Work out the finished part from the listing and answer in its coordinate system (mm). A direction names the side the tool comes from. Round coordinates to 2 decimals unless told otherwise and drop trailing zeros. Loops run counter-clockwise (first coordinate to the right, second up) from the corner with the lowest first, then second, coordinate; pieces in that order, holes last. Notation, with made-up numbers: (-30.75, -40) -> (14.25, -40) arc R11 cw to (14.25, -23) -> close; hole circle Ø1 at (1.25, -37.5). An arc over 180 degrees is marked (long way). Use one line per item in the form item = value.
```python
from build123d import *

# Parameters (mm, degrees)
SKICA2_W                 = 20
SKICA2_H                 = 42.3
P_IDAT_VYSUNUT_M1_DEPTH  = 4
SKICA3_W                 = 24
SKICA3_H                 = 42.3
P_IDAT_VYSUNUT_M2_DEPTH  = 4
SKICA4_W                 = 6
SKICA4_H                 = 42.3
P_IDAT_VYSUNUT_M3_DEPTH  = 42.3
SKICA5_R                 = 11.05
ODEBRAT_VYSUNUT_M1_DEPTH = 7
SKICA7_R                 = 2.6
ODEBRAT_VYSUNUT_M3_DEPTH = 4
ZKOSEN_1_SIZE            = 1
SKICA8_W                 = 20
SKICA8_H                 = 4
P_IDAT_VYSUNUT_M4_DEPTH  = 20.091596743
SKICA9_R                 = 2.6
ODEBRAT_VYSUNUT_M4_DEPTH = 4
ODEBRAT_VYSUNUT_M5_DEPTH = 80
SKICA11_W                = 84.692176523
SKICA11_H                = 80.474242756
ODEBRAT_VYSUNUT_M6_DEPTH = 24
SKICA12_W                = 6
SKICA12_H                = 6
SKICA12_H_2              = 10
P_IDAT_VYSUNUT_M5_DEPTH  = 8
SKICA13_R                = 1.6
ODEBRAT_VYSUNUT_M7_DEPTH = 15
SKICA14_W                = 5
SKICA14_H                = 3
ODEBRAT_VYSUNUT_M8_DEPTH = 15


with BuildPart() as part:
    # Skica2 → Přidat vysunutím1 (new body)
    with BuildSketch(Plane.XY):
        with Locations((-14.524287798, -61.15)):
            Rectangle(SKICA2_W, SKICA2_H)
    extrude(amount=P_IDAT_VYSUNUT_M1_DEPTH)

    # Skica3 → Přidat vysunutím2 (add)
    with BuildSketch(Plane.ZY.offset(24.524287798)):
        with Locations((-8, -61.15)):
            Rectangle(SKICA3_W, SKICA3_H)
    extrude(amount=P_IDAT_VYSUNUT_M2_DEPTH)

    # Skica4 → Přidat vysunutím3 (add)
    with BuildSketch(Plane.XY.offset(4)):
        with Locations((-7.524287798, -61.15)):
            Rectangle(SKICA4_W, SKICA4_H)
    extrude(amount=P_IDAT_VYSUNUT_M3_DEPTH)

    # Skica5 → Odebrat vysunutím1 (cut)
    with BuildSketch(Plane(origin=(-4.524287798, 0, 0), x_dir=(0, 0, -1), z_dir=(1, 0, 0))):
        with Locations((-25.15, -61.15)):
            Circle(SKICA5_R)
    extrude(amount=-ODEBRAT_VYSUNUT_M1_DEPTH, mode=Mode.SUBTRACT)

    # Skica7 → Odebrat vysunutím3 (cut)
    with BuildSketch(Plane.ZY.offset(28.524287798)):
        with Locations(Location((-10, -50, 0), (0, 0, 270))):
            Circle(SKICA7_R)
        with Locations(Location((-10, -70, 0), (0, 0, 270))):
            Circle(SKICA7_R)
    extrude(amount=-ODEBRAT_VYSUNUT_M3_DEPTH, mode=Mode.SUBTRACT)

    # Zkosení1
    zkosen_1_edges = [part.edges().sort_by_distance(p)[0] for p in [
        (-10.524287798, -61.15, 36.2),
    ]]
    chamfer(zkosen_1_edges, length=ZKOSEN_1_SIZE)

    # Skica8 → Přidat vysunutím4 (add)
    with BuildSketch(Plane.XZ.offset(82.3)):
        with Locations((-14.524287798, 2)):
            Rectangle(SKICA8_W, SKICA8_H)
    extrude(amount=P_IDAT_VYSUNUT_M4_DEPTH)

    # Skica9 → Odebrat vysunutím4 (cut)
    with BuildSketch(Plane.XY.offset(4)):
        with Locations((-14.524287798, -92.391596743)):
            Circle(SKICA9_R)
    extrude(amount=-ODEBRAT_VYSUNUT_M4_DEPTH, mode=Mode.SUBTRACT)

    # Skica10 → Odebrat vysunutím5 (cut)
    with BuildSketch(Plane.ZY.offset(10.524287798)):
        Polygon((46.3, -44), (42.3, -40), (46.565878614, -39.259270079), align=None)
        Polygon((42.3, -82.3), (46.3, -78.3), (47.745576453, -80.3), (46.3, -85.415433185), align=None)
    extrude(amount=-ODEBRAT_VYSUNUT_M5_DEPTH, mode=Mode.SUBTRACT)


with BuildPart() as body_2:
    # Zrcadlit1: mirrored copy
    add(part.part.mirror(Plane(origin=(-28.524287798, -40, -20), x_dir=(1, 0, 0), z_dir=(0, 0, 1))))

    # Skica12 → Přidat vysunutím5 (add)
    with BuildSketch(Plane(origin=(0, -40, 0), x_dir=(1, 0, 0), z_dir=(0, 1, 0))):
        with Locations((-7.524287798, 79.3)):
            Rectangle(SKICA12_W, SKICA12_H)
        with Locations((-7.524287798, 59.3)):
            Rectangle(SKICA12_W, SKICA12_H_2)
    extrude(amount=P_IDAT_VYSUNUT_M5_DEPTH)

    # Skica13 → Odebrat vysunutím7 (cut)
    with BuildSketch(Plane(origin=(0, -32, 0), x_dir=(1, 0, 0), z_dir=(0, 1, 0))):
        with Locations(Location((-7.524287798, 59.3, 0), (0, 0, 270))):
            Circle(SKICA13_R)
        with Locations(Location((-7.524287798, 79.3, 0), (0, 0, 270))):
            Circle(SKICA13_R)
    extrude(amount=-ODEBRAT_VYSUNUT_M7_DEPTH, mode=Mode.SUBTRACT)

    # Skica14 → Odebrat vysunutím8 (cut)
    with BuildSketch(Plane(origin=(-4.524287798, 0, 0), x_dir=(0, 0, -1), z_dir=(1, 0, 0))):
        with Locations((59.3, -44.438988808)):
            Rectangle(SKICA14_W, SKICA14_H)
        with Locations((79.3, -44.438988808)):
            Rectangle(SKICA14_W, SKICA14_H)
    extrude(amount=-ODEBRAT_VYSUNUT_M8_DEPTH, mode=Mode.SUBTRACT)


with BuildPart() as part_1:
    add(part.part)

    # Skica11 → Odebrat vysunutím6 (cut)
    with BuildSketch(Plane.ZY.offset(28.524287798)):
        with Locations((22.346088262, -80.237121378)):
            Rectangle(SKICA11_W, SKICA11_H)
    extrude(amount=-ODEBRAT_VYSUNUT_M6_DEPTH, mode=Mode.SUBTRACT)


solid = body_2.part
```
(1) Find section A-A, the plane z = -65.15. Write down the section's boundary in (x, y).
Completed:
outline = (-10.52, -82.3) -> (-4.52, -82.3) -> (-4.52, -72.2) -> (-9.52, -72.2) -> (-10.52, -73.2) -> close; (-10.52, -49.1) -> (-9.52, -50.1) -> (-4.52, -50.1) -> (-4.52, -40) -> (-10.52, -40) -> close
(2) Find section D-D, the plane z = -79.3. Write down the section's boundary in (x, y), then the cut area to 3 significant figures.
Completed:
outline = (-10.52, -82.3) -> (-4.52, -82.3) -> (-4.52, -45.94) -> (-5.92, -45.94) -> (-5.92, -47) -> (-9.12, -47) -> (-9.12, -45.94) -> (-10.52, -45.94) -> close; (-10.52, -42.94) -> (-9.12, -42.94) -> (-9.12, -32) -> (-10.52, -32) -> close; (-5.92, -42.94) -> (-4.52, -42.94) -> (-4.52, -32) -> (-5.92, -32) -> close
area = 245 mm2
(3) Given P1, Ø5, axis at x = -6.5, z = -67.5, coming from the +Y side; P2, Ø12.5, axis at y = -46.5, z = -64.5, coming from the -X side; P3, Ø10, axis at y = -90, z = -41, coming from the -X side, each flat-ended and moving along its own axis, determine where each tip first touches the part or whether it passes through.
Completed:
P1 = -40
P2 = -10.52
P3 = -24.52
(4) Find section C-C, the plane x = -26. Write down the section's boundary in (y, z), then the cut area to 3 significant figures.
Completed:
outline = (-82.3, -44) -> (-40, -44) -> (-40, -20) -> (-82.3, -20) -> close; hole circle Ø5.2 at (-70, -30); hole circle Ø5.2 at (-50, -30)
area = 973 mm2
(5) Find section B-B, the plane y = -61.15. Write down the section's boundary in (x, z), then the cut area to 3 significant figures.
Completed:
outline = (-28.52, -44) -> (-10.52, -44) -> (-10.52, -53.1) -> (-9.52, -54.1) -> (-4.52, -54.1) -> (-4.52, -40) -> (-24.52, -40) -> (-24.52, -20) -> (-28.52, -20) -> close; (-10.52, -86.3) -> (-4.52, -86.3) -> (-4.52, -76.2) -> (-9.52, -76.2) -> (-10.52, -77.2) -> close
area = 296 mm2
(6) Consider L1, parallel to Z at x = -7.75, y = -43; L2, parallel to Z at x = -25.4, y = -70; L3, parallel to Y at x = -7.4, z = -65.15. Determine where each line is inside the solid, lowest interval first.
Completed:
L1 = -85.3 to -81.8, -76.8 to -61.8, -56.8 to -40
L2 = -44 to -32.6, -27.4 to -20
L3 = -82.3 to -72.2, -50.1 to -40
(7) For faces 1 (the flat face through (-8, -40, -70)), 2 (the flat face through (-8, -82.3, -63)), 3 (the flat face through (-15, -71, -40)), 4 (the flat face through (-7, -45.939, -61)), determine the directions among +Z, -Z, +X, -X, +Y, -Y from which every point of the face is accessible in a straight line to the end or side of a thin tool.
Completed:
face_1 = +X, -X, +Y
face_2 = -Z, +X, -X, -Y
face_3 = +Z, +X, +Y, -Y
face_4 = +X, -X
(8) For a pull along Y with two mould halves and no side action, classify faces 5 (the flat face through (-7, -42.939, -61)), 6 (the flat face through (-8, -47, -59)), 7 (the flat face through (-8, -36, -64.3)) as +Y half, -Y half, draft (parallel to the pull), parting line (faces both ways), or undercut.
Completed:
face_5 = undercut
face_6 = +Y half
face_7 = draft
